Verification items for the finished model (mm, model axes). Coordinates: 2 decimals unless noted, no trailing zeros. Order: outer loops, then holes, each group sorted by start corner. A loop starts at its lowest first (then second) coordinate and runs counter-clockwise, first axis right, second up. Notation, with made-up numbers: (62.5, -29) -> (97.5, -29) arc R12 ccw to (97.5, -18) -> close; hole circle Ø9 at (47.25, 58.25). An arc over 180 degrees is marked (long way). Answer as CSV lines item,"result".
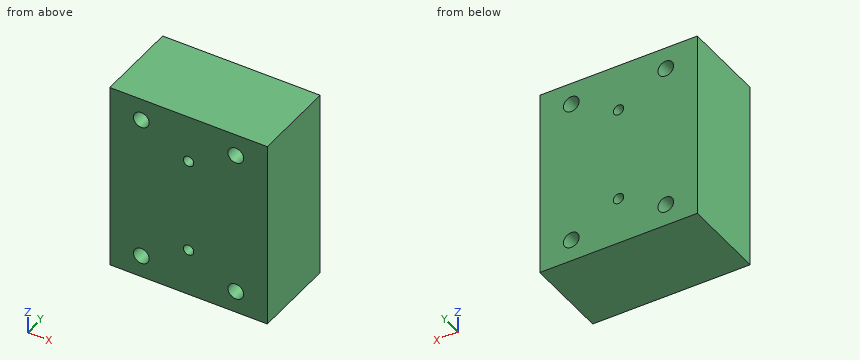
```python
from build123d import *

# Parameters (mm, degrees)
SKETCH_1_W             = 50
SKETCH_1_H             = 27
EXTRUDE_1_DEPTH        = 60
SKETCH_2_R             = 2.5
CUT_EXTRUDE_1_DEPTH    = 27
PATTERN_LINEAR_1_COUNT = 2
PATTERN_LINEAR_1_PITCH = 46
SKETCH_3_R             = 2.5
CUT_EXTRUDE_2_DEPTH    = 27
PATTERN_LINEAR_2_COUNT = 2
PATTERN_LINEAR_2_PITCH = 46
SKETCH_4_R             = 1.65
CUT_EXTRUDE_3_DEPTH    = 27


with BuildPart() as part:
    # Эскиз1 → Бобышка-Вытянуть1 (new body)
    with BuildSketch(Plane.XY):
        Rectangle(SKETCH_1_W, SKETCH_1_H)
    extrude(amount=EXTRUDE_1_DEPTH)

    # Эскиз2 → Вырез-Вытянуть1 (cut)
    with BuildSketch(Plane(origin=(0, 13.5, 0), x_dir=(1, 0, 0), z_dir=(0, 1, 0))):
        with Locations(Location((-15, -7, 0), (0, 0, 180))):
            Circle(SKETCH_2_R)
    cut_extrude_1 = extrude(amount=-CUT_EXTRUDE_1_DEPTH, mode=Mode.SUBTRACT)

    # Линейный массив1: Вырез-Вытянуть1 ×2
    with Locations(*[(0, 0, i * PATTERN_LINEAR_1_PITCH) for i in range(1, PATTERN_LINEAR_1_COUNT)]):
        add(cut_extrude_1, mode=Mode.SUBTRACT)

    # Эскиз3 → Вырез-Вытянуть2 (cut)
    with BuildSketch(Plane(origin=(0, 13.5, 0), x_dir=(1, 0, 0), z_dir=(0, 1, 0))):
        with Locations(Location((15, -7, 0), (0, 0, 180))):
            Circle(SKETCH_3_R)
    cut_extrude_2 = extrude(amount=-CUT_EXTRUDE_2_DEPTH, mode=Mode.SUBTRACT)

    # Линейный массив2: Вырез-Вытянуть2 ×2
    with Locations(*[(0, 0, i * PATTERN_LINEAR_2_PITCH) for i in range(1, PATTERN_LINEAR_2_COUNT)]):
        add(cut_extrude_2, mode=Mode.SUBTRACT)

    # Эскиз4 → Вырез-Вытянуть3 (cut)
    with BuildSketch(Plane(origin=(0, 13.5, 0), x_dir=(1, 0, 0), z_dir=(0, 1, 0))):
        with Locations(Location((0, -15, 0), (0, 0, 270))):
            Circle(SKETCH_4_R)
        with Locations(Location((0, -45, 0), (0, 0, 270))):
            Circle(SKETCH_4_R)
    extrude(amount=-CUT_EXTRUDE_3_DEPTH, mode=Mode.SUBTRACT)


solid = part.part
```
Item 1: Section check D-D, the plane y = 1.25. Record the boundary of the cut face in (x, z).
Answer list:
outline,"(-25, 0) -> (25, 0) -> (25, 60) -> (-25, 60) -> close; hole circle Ø5 at (-15, 7); hole circle Ø5 at (-15, 53); hole circle Ø3.3 at (0, 15); hole circle Ø3.3 at (0, 45); hole circle Ø5 at (15, 7); hole circle Ø5 at (15, 53)"
Item 2: Section check C-C, the plane z = 15. Record the boundary of the cut face in (x, y), plus the area to 3 significant figures.
Answer list:
outline,"(-25, -13.5) -> (-1.65, -13.5) -> (-1.65, 13.5) -> (-25, 13.5) -> close; (1.65, -13.5) -> (25, -13.5) -> (25, 13.5) -> (1.65, 13.5) -> close"
area,"1,260 mm2"
Item 3: Section check B-B, the plane z = 53. Record the boundary of the cut face in (x, y).
Answer list:
outline,"(-25, -13.5) -> (-17.5, -13.5) -> (-17.5, 13.5) -> (-25, 13.5) -> close; (-12.5, -13.5) -> (12.5, -13.5) -> (12.5, 13.5) -> (-12.5, 13.5) -> close; (17.5, -13.5) -> (25, -13.5) -> (25, 13.5) -> (17.5, 13.5) -> close"
Item 4: Depth check by flat-ended pin: pin 1 Ø4 at (x, y) = (11, 6.5) entering from -Z; pin 2 Ø4 at (x, z) = (15, 7) entering from -Y. Enter the tip coordinate at first touch or a pass-through.
Answer list:
pin 1,"z = 0"
pin 2,"through"
Item 5: Section check A-A, the plane x = 0. Record the boundary of the cut face in (y, z), plus the area to 3 significant figures.
Answer list:
outline,"(-13.5, 0) -> (13.5, 0) -> (13.5, 13.35) -> (-13.5, 13.35) -> close; (-13.5, 16.65) -> (13.5, 16.65) -> (13.5, 43.35) -> (-13.5, 43.35) -> close; (-13.5, 46.65) -> (13.5, 46.65) -> (13.5, 60) -> (-13.5, 60) -> close"
area,"1,440 mm2"
Item 6: Thickness scan on line 1 (Z direction, x = 15, y = -7.5); line 2 (X direction, y = -7.25, z = 45); line 3 (Z direction, x = -1, y = -7.5). Record the ranges inside material, lowest first.
Answer list:
line 1,"0 to 4.5, 9.5 to 50.5, 55.5 to 60"
line 2,"-25 to -1.65, 1.65 to 25"
line 3,"0 to 13.69, 16.31 to 43.69, 46.31 to 60"
